Check sheet for the modelled part. Datum: model origin and axes. Units: mm. Face numbers are marked on the shaded views. A direction names the side the tool comes from. Round coordinates to 2 decimals unless told otherwise and drop trailing zeros. Order: outer loops, then holes, each group sorted by start corner. A loop starts at its lowest first (then second) coordinate and runs counter-clockwise, first axis right, second up.
(1) Sectioned sample at A-A, the plane x = 8.89. Enter the section's corners in (y, z) (3 decimals).
(2) Sectioned sample at C-C, the plane z = 6. Enter the section's corners in (x, y), and give its area (3 significant figures).
(3) Tool access check on the marked faces 4, 5, 6, 7 and 8. Record the directions out of +Z, -Z, +X, -X, +Y, -Y that give a thin tool (end or side, any length) a straight path to the whole face; none if there is none.
(4) Depth check by flat-ended pin: pin 1 (6 mm diameter, centred on x = 9, y = 50, fed in from +Z) (3 decimals); pin 2 (1 mm diameter, centred on y = 35.5, z = 13, fed in from +X); pin 3 (8 mm diameter, centred on x = -24, z = 7.5, fed in from -Y). Enter the tip coordinate at first touch or a pass-through.
(5) Sectioned sample at D-D, the plane x = -20.5. Enter the section's corners in (y, z) (3 decimals).
(6) Thickness scan on probe 1 along X at (y, z) = (-8.89, 2.2); probe 2 along X at (y, z) = (50.8, 1.45); probe 3 along Y at (x, z) = (-38, 2.5). Record the ranges inside material, lowest first.
(7) Mould release check, pull along X, two halves, no side actions. Record for the marked faces 1, 2 and 3: released by +X, released by -X, zero draft, split by the parting line, or undercut.
(8) Sectioned sample at B-B, the plane y = -8.89. Enter the section's corners in (x, z) (3 decimals).
```python
from build123d import *

# Parameters (mm, degrees)
SKETCH2_W                                   = 54.61
SKETCH2_H                                   = 41.91
SKETCH2_W_2                                 = 41.91
SKETCH2_H_2                                 = 29.21
BOSS_EXTRUDE1_DEPTH                         = 9.525
SKETCH4_W                                   = 41.91
SKETCH4_H                                   = 54.61
BOSS_EXTRUDE2_DEPTH                         = 6.35
SKETCH6_R                                   = 3.2004
CUT_EXTRUDE1_DEPTH                          = 63.012553769
SKETCH7_W                                   = 67.31
SKETCH7_H                                   = 54.61
SKETCH7_W_2                                 = 54.61
SKETCH7_H_2                                 = 41.91
BOSS_EXTRUDE3_DEPTH                         = 3.175
CBORE_FOR_2_BINDING_HEAD_MACHINE_SC_2_COUNT = 2
CBORE_FOR_2_BINDING_HEAD_MACHINE_SC_2_PITCH = 46.99
CBORE_FOR_2_BINDING_HEAD_MACHINE_SC_3_COUNT = 2
CBORE_FOR_2_BINDING_HEAD_MACHINE_SC_3_PITCH = 75.966809858
CBORE_FOR_2_BINDING_HEAD_MACHINE_SC_4_COUNT = 2
CBORE_FOR_2_BINDING_HEAD_MACHINE_SC_4_PITCH = 59.69
FILLET1_R                                   = 1.27


with BuildPart() as part:
    # Sketch2 → Boss-Extrude1 (new body)
    with BuildSketch(Plane(origin=(0, 0, 0), x_dir=(0, 1, 0), z_dir=(0, 0, 1))):
        with Locations((20.955, 14.605)):
            Rectangle(SKETCH2_W, SKETCH2_H)
        with Locations((20.955, 14.605)):
            Rectangle(SKETCH2_W_2, SKETCH2_H_2, mode=Mode.SUBTRACT)
    extrude(amount=BOSS_EXTRUDE1_DEPTH)

    # Sketch4 → Boss-Extrude2 (add)
    with BuildSketch(Plane.XY.offset(9.525)):
        with Locations((-14.605, 20.955)):
            Rectangle(SKETCH4_W, SKETCH4_H)
    extrude(amount=BOSS_EXTRUDE2_DEPTH)

    # Sketch6 → Cut-Extrude1 (cut, through all)
    with BuildSketch(Plane.XY.offset(15.875)):
        with Locations((-14.605, 10.668)):
            Circle(SKETCH6_R)
    extrude(amount=-CUT_EXTRUDE1_DEPTH, mode=Mode.SUBTRACT)

    # Sketch7 → Boss-Extrude3 (add)
    with BuildSketch(Plane(origin=(0, 0, 0), x_dir=(0, 1, 0), z_dir=(0, 0, 1))):
        with Locations((20.955, 14.605)):
            Rectangle(SKETCH7_W, SKETCH7_H)
        with Locations((20.955, 14.605)):
            Rectangle(SKETCH7_W_2, SKETCH7_H_2, mode=Mode.SUBTRACT)
    extrude(amount=BOSS_EXTRUDE3_DEPTH)

    # Sketch9 → CBORE for #2 Binding Head Machine Screw1 (revolve, cut)
    with BuildSketch(Plane(origin=(-38.1, 50.8, 3.175), x_dir=(0, -1, 0), z_dir=(1, 0, 0))):
        Polygon((0, 0), (0, 3.175), (1.2954, 3.175), (1.2954, 1.27), (2.77876, 1.27), (2.77876, 0.635), (3.41376, 0), align=None)
    cbore_for_2_binding_head_machine_screw1 = revolve(axis=Axis((-38.1, 50.8, 9.525), (0, 0, -1)), mode=Mode.SUBTRACT)

    # CBORE for _2 Binding Head Machine Sc 2: CBORE for #2 Binding Head Machine Screw1 ×2
    with Locations(*[(i * CBORE_FOR_2_BINDING_HEAD_MACHINE_SC_2_PITCH, 0, 0) for i in range(1, CBORE_FOR_2_BINDING_HEAD_MACHINE_SC_2_COUNT)]):
        add(cbore_for_2_binding_head_machine_screw1, mode=Mode.SUBTRACT)

    # CBORE for _2 Binding Head Machine Sc 3: CBORE for #2 Binding Head Machine Screw1 ×2
    with Locations(*[Vector(0.6185596063312605, -0.7857378783126826, 0) * (i * CBORE_FOR_2_BINDING_HEAD_MACHINE_SC_3_PITCH) for i in range(1, CBORE_FOR_2_BINDING_HEAD_MACHINE_SC_3_COUNT)]):
        add(cbore_for_2_binding_head_machine_screw1, mode=Mode.SUBTRACT)

    # CBORE for _2 Binding Head Machine Sc 4: CBORE for #2 Binding Head Machine Screw1 ×2
    with Locations(*[(0, -i * CBORE_FOR_2_BINDING_HEAD_MACHINE_SC_4_PITCH, 0) for i in range(1, CBORE_FOR_2_BINDING_HEAD_MACHINE_SC_4_COUNT)]):
        add(cbore_for_2_binding_head_machine_screw1, mode=Mode.SUBTRACT)

    # Fillet1
    fillet1_edges = [part.edges().sort_by_distance(p)[0] for p in [
        (-35.56, 20.955, 15.875),
        (-14.605, -6.35, 15.875),
        (6.35, 20.955, 15.875),
        (-14.605, 48.26, 15.875),
        (-41.91, -12.7, 1.5875),
        (12.7, -12.7, 1.5875),
        (12.7, 54.61, 1.5875),
        (-41.91, 54.61, 1.5875),
        (-35.56, -6.35, 9.525),
        (-35.56, 48.26, 9.525),
        (6.35, 48.26, 9.525),
        (6.35, -6.35, 9.525),
    ]]
    fillet(fillet1_edges, radius=FILLET1_R)


solid = part.part
```
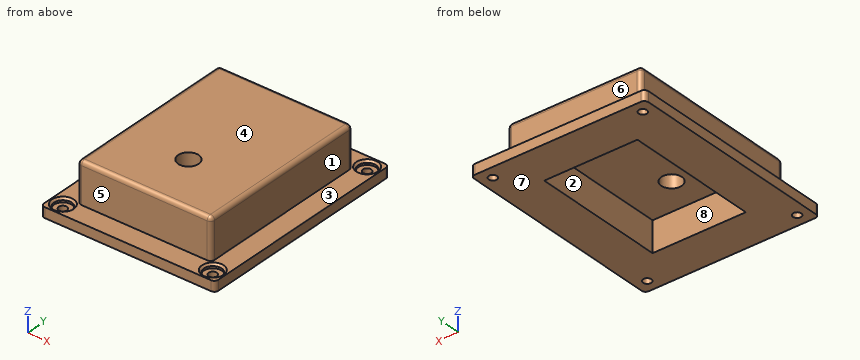
Derived:
1. outline: (-12.7, 0) - (-10.185, 0) - (-10.185, 1.905) - (-11.669, 1.905) - (-11.669, 2.54) - (-12.304, 3.175) - (-12.7, 3.175) - close; (-7.595, 0) - (49.505, 0) - (49.505, 1.905) - (48.021, 1.905) - (48.021, 2.54) - (47.386, 3.175) - (-5.476, 3.175) - (-6.111, 2.54) - (-6.111, 1.905) - (-7.595, 1.905) - close; (52.095, 0) - (54.61, 0) - (54.61, 3.175) - (54.214, 3.175) - (53.579, 2.54) - (53.579, 1.905) - (52.095, 1.905) - close
2. outline: (-35.56, -5.08) arc R1.27 ccw to (-34.29, -6.35) - (5.08, -6.35) arc R1.27 ccw to (6.35, -5.08) - (6.35, 46.99) arc R1.27 ccw to (5.08, 48.26) - (-34.29, 48.26) arc R1.27 ccw to (-35.56, 46.99) - close; hole (-29.21, 0) - (0, 0) - (0, 41.91) - (-29.21, 41.91) - close
2. area: 1,060 mm2
3. face 4: +Z, +X, -X, +Y, -Y
3. face 5: +Z, +X, -X, -Y
3. face 6: +Z, +X, -X, +Y
3. face 7: -Z, +X, -X, +Y, -Y
3. face 8: -Z
4. pin 1: stops at z = 3.175
4. pin 2: stops at x = 6.35
4. pin 3: stops at y = -6.35
5. outline: (-12.7, 0) - (0, 0) - (0, 9.525) - (41.91, 9.525) - (41.91, 0) - (54.61, 0) - (54.61, 3.175) - (48.26, 3.175) - (48.26, 14.605) arc R1.27 ccw to (46.99, 15.875) - (-5.08, 15.875) arc R1.27 ccw to (-6.35, 14.605) - (-6.35, 3.175) - (-12.7, 3.175) - close
6. probe 1: x = -41.91 to -40.88, -35.32 to 6.11, 11.67 to 12.7
6. probe 2: x = -41.91 to -39.4, -36.8 to 7.59, 10.19 to 12.7
6. probe 3: y = -12.7 to -11.67, -6.11 to 48.02, 53.58 to 54.61
7. face 1: released by +X
7. face 2: undercut
7. face 3: zero draft
8. outline: (-41.91, 0) - (-39.395, 0) - (-39.395, 1.905) - (-40.879, 1.905) - (-40.879, 2.54) - (-41.514, 3.175) - (-41.91, 3.175) - close; (-36.805, 0) - (7.595, 0) - (7.595, 1.905) - (6.111, 1.905) - (6.111, 2.54) - (5.476, 3.175) - (-34.686, 3.175) - (-35.321, 2.54) - (-35.321, 1.905) - (-36.805, 1.905) - close; (10.185, 0) - (12.7, 0) - (12.7, 3.175) - (12.304, 3.175) - (11.669, 2.54) - (11.669, 1.905) - (10.185, 1.905) - close
